```python
from build123d import *

# Parameters (mm, degrees)
F1_DEPTH = 20
F2_DEPTH = 20
F3_W     = 15.387754
F3_H     = 7.40892
F4_DEPTH = 50
F5_R     = 1
F6_R     = 1


with BuildPart() as f1:
    # F0 (on Front) → F1 (new body)
    with BuildSketch(Plane.XZ):
        with BuildLine():
            ThreePointArc((35.22866, 13.946989), (35.556946, 11.245402), (37.857051, 12.7))
            ThreePointArc((37.857051, 12.7), (36.937157, 14.154598), (35.22866, 13.946989))
        make_face()
    extrude(amount=F1_DEPTH)

    # F0 (on Front) → F2 (join)
    with BuildSketch(Plane.XZ):
        with BuildLine():
            Line((22.057051, 3.19), (22.057051, 0))
            Line((22.057051, 0), (37.857051, 0))
            Line((37.857051, 0), (37.857051, 12.7))
            ThreePointArc((37.857051, 12.7), (35.556946, 11.245402), (35.22866, 13.946989))
            Line((35.22866, 13.946989), (22.057051, 3.19))
        make_face()
        with BuildLine():
            ThreePointArc((35.22866, 13.946989), (35.556946, 11.245402), (37.857051, 12.7))
            ThreePointArc((37.857051, 12.7), (36.937157, 14.154598), (35.22866, 13.946989))
        make_face()
    extrude(amount=F2_DEPTH)

    # F3 (on Right) → F4 (cut)
    with BuildSketch(Plane.YZ):
        with Locations((-9.89757, 7.296514)):
            Rectangle(F3_W, F3_H)
    extrude(amount=F4_DEPTH, mode=Mode.SUBTRACT)

    # F5
    f5_edges = [f1.edges().sort_by_distance(p)[0] for p in [
        (31.621354, -9.89757, 11.000974),
    ]]
    fillet(f5_edges, radius=F5_R)

    # F6
    f6_edges = [f1.edges().sort_by_distance(p)[0] for p in [
        (37.857051, -9.89757, 11.000974),
    ]]
    fillet(f6_edges, radius=F6_R)


solid = f1.part
```
Geometry check sheet. Reference: the model listing, model coordinates, mm. A direction names the side the tool comes from. Round coordinates to 2 decimals unless told otherwise and drop trailing zeros. Loops run counter-clockwise (first coordinate to the right, second up) from the corner with the lowest first, then second, coordinate; pieces in that order, holes last. Notation, with made-up numbers: (-21.75, 40.25) - (22.25, 40.25) arc R20 cw to (22.25, 63.25) - close; hole circle Ø4 at (6.25, 15). An arc over 180 degrees is marked (long way). Use a Markdown table: item, result.
Q1. Cross-section at B-B on x = 36.5. Record the cut outline in (y, z).
Solutions:
| item | result |
|---|---|
| outline | (-20, 0) - (0, 0) - (0, 14.29) - (-20, 14.29) - close; hole (-17.59, 3.59) - (-2.2, 3.59) - (-2.2, 11) - (-17.59, 11) - close |
Q2. Cross-section at C-C on y = -1.25. Record the cut outline in (x, z).
Solutions:
| item | result |
|---|---|
| outline | (22.06, 0) - (37.86, 0) - (37.86, 12.7) arc R1.61 ccw to (35.23, 13.95) - (22.06, 3.19) - close |
Q3. Cross-section at D-D on x = 30.5. Record the cut outline in (y, z).
Solutions:
| item | result |
|---|---|
| outline | (-20, 0) - (0, 0) - (0, 10.09) - (-2.2, 10.09) - (-2.2, 3.59) - (-17.59, 3.59) - (-17.59, 10.09) - (-20, 10.09) - close |
Q4. Draft check along Z on faces 4 (the flat face through (30, -10, 0)), 5 (the cylindrical face through (33.48, -10.01, 11.68)), 6 (the flat face through (32, 0, 6)). Enter one of: released by +Z, released by -Z, zero draft, split by the parting line, or undercut.
Solutions:
| item | result |
|---|---|
| face 4 | released by -Z |
| face 5 | undercut |
| face 6 | zero draft |
Q5. Cross-section at A-A on z = 4.75. Record the cut outline in (x, y), plus the area to 3 significant figures.
Solutions:
| item | result |
|---|---|
| outline | (23.97, -20) - (37.86, -20) - (37.86, -17.59) - (23.97, -17.59) - close; (23.97, -2.2) - (37.86, -2.2) - (37.86, 0) - (23.97, 0) - close |
| area | 64.1 mm2 |
Q6. Go/stop test with flat-tipped pins: P1, Ø6, axis at y = -9.5, z = 8.5, coming from the +X side; P2, Ø1, axis at x = 24.5, y = -11.5, coming from the +Z side; P3, Ø2.5, axis at x = 36, y = -9.5, coming from the -Z side; P4, Ø1, axis at y = -17.5, z = 5.5, coming from the -X side. Record where each tip stops, or that it passes through.
Solutions:
| item | result |
|---|---|
| P1 | stops at x = 37.72 |
| P2 | stops at z = 3.59 |
| P3 | stops at z = 0 |
| P4 | stops at x = 24.28 |
Q7. Access from +Z, -Z, +X, -X, +Y, -Y to the whole of each face (thin tool, end or side, straight path). Record for faces 1 (the cylindrical face through (37.57, -9.79, 11.3)), 2 (the flat face through (34.04, -10.694, 12.976)), 3 (the flat face through (30, -10, 3.592)).
Solutions:
| item | result |
|---|---|
| face 1 | +X |
| face 2 | +Z, -X, +Y, -Y |
| face 3 | +X, -X |
Q8. Material ranges on line 1 (Y direction, x = 26.75, z = 4.75); line 2 (X direction, y = -15.25, z = 12); line 3 (Z direction, x = 22.75, y = -15), recorded low to high.
Solutions:
| item | result |
|---|---|
| line 1 | y = -20 to -17.59, -2.2 to 0 |
| line 2 | x = 33.43 to 37.86 |
| line 3 | z = 0 to 3.59 |
